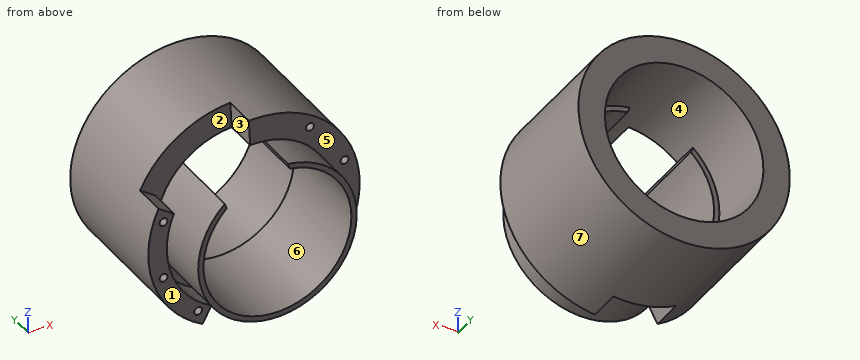
```python
from build123d import *

# Parameters (mm, degrees)
ESBO_O1_R                     = 40
ESBO_O1_R_2                   = 30
RESSALTO_EXTRUS_O1_DEPTH      = 50
ESBO_O2_R                     = 1.5
CORTE_EXTRUS_O1_DEPTH         = 10
CORTE_EXTRUS_O2_DEPTH         = 11.84997677
RESSALTO_EXTRUS_O2_DEPTH      = 26.84997677
RESSALTO_EXTRUS_O2_DEPTH_BACK = 10
ESCALA1_SCALE                 = 0.681818182


with BuildPart() as part:
    # Esboço1 → Ressalto-extrusão1 (new body)
    with BuildSketch(Plane(origin=(0, 0, 0), x_dir=(1, 0, 0), z_dir=(0, 1, 0))):
        with Locations(Location((0, 0, 0), (0, 0, 270))):
            Circle(ESBO_O1_R)
        with Locations(Location((0, 0, 0), (0, 0, 270))):
            Circle(ESBO_O1_R_2, mode=Mode.SUBTRACT)
    extrude(amount=RESSALTO_EXTRUS_O1_DEPTH)

    # Esboço2 → Corte-extrusão1 (cut)
    with BuildSketch(Plane(origin=(0, 0, 0), x_dir=(-1, 0, 0), z_dir=(0, -1, 0))):
        with Locations(Location((-21.160269083, -29.124611797, 0), (0, 0, 90))):
            Circle(ESBO_O2_R)
        with Locations(Location((-34.238034587, -11.124611797, 0), (0, 0, 90))):
            Circle(ESBO_O2_R)
        with Locations(Location((-34.238034587, 11.124611797, 0), (0, 0, 90))):
            Circle(ESBO_O2_R)
        with Locations(Location((21.160269083, 29.124611797, 0), (0, 0, 90))):
            Circle(ESBO_O2_R)
        with Locations(Location((34.238034587, 11.124611797, 0), (0, 0, 90))):
            Circle(ESBO_O2_R)
        with Locations(Location((34.238034587, -11.124611797, 0), (0, 0, 90))):
            Circle(ESBO_O2_R)
    extrude(amount=-CORTE_EXTRUS_O1_DEPTH, mode=Mode.SUBTRACT)

    # Esboço3 → Corte-extrusão2 (cut)
    with BuildSketch(Plane(origin=(0, 0, 0), x_dir=(-1, 0, 0), z_dir=(0, -1, 0))):
        with BuildLine():
            ThreePointArc((30.293924668, -13.087327008), (31.253408489, 10.593604572), (16.092357529, 28.81034587))
            Line((16.092357529, 28.81034587), (19.505887914, 34.921631358))
            ThreePointArc((19.505887914, 34.921631358), (8.030354378, 39.185627576), (-4.197370073, 39.779166463))
            Line((-4.197370073, 39.779166463), (-3.148027555, 29.834374847))
            ThreePointArc((-3.148027555, 29.834374847), (29.911212101, 2.306380417), (1.462902849, -29.964310692))
            Line((1.462902849, -29.964310692), (1.950537132, -39.952414256))
            ThreePointArc((1.950537132, -39.952414256), (22.185986252, -33.283359416), (36.126859334, -17.171197823))
            Line((36.126859334, -17.171197823), (30.293924668, -13.087327008))
        make_face()
    extrude(amount=-CORTE_EXTRUS_O2_DEPTH, mode=Mode.SUBTRACT)

    # Esboço4 → Ressalto-extrusão2 (add, two sides: drawn at the far end of the back side and taken through both)
    with BuildSketch(Plane(origin=(0, 11.84997677, 0), x_dir=(-1, 0, 0), z_dir=(0, -1, 0)).offset(-RESSALTO_EXTRUS_O2_DEPTH_BACK)):
        with BuildLine():
            Line((-4.008838629, -29.730947056), (-4.700362463, -27.602655537))
            ThreePointArc((-4.700362463, -27.602655537), (-8.119302432, 26.79695744), (19.230258499, -20.351834268))
            Line((19.230258499, -20.351834268), (19.909240802, -22.441526924))
            ThreePointArc((19.909240802, -22.441526924), (-8.745833796, 28.696870757), (-4.008838629, -29.730947056))
        make_face()
    extrude(amount=RESSALTO_EXTRUS_O2_DEPTH + RESSALTO_EXTRUS_O2_DEPTH_BACK)


with BuildPart() as part_1:
    # Escala1: scaled about (0, 0, 0)
    add(part.part.scale(ESCALA1_SCALE))


solid = part_1.part
```
Geometry check sheet. Reference: the model listing, model coordinates, mm. Face numbers are marked on the shaded views. A direction names the side the tool comes from. Give positions to 0.01 mm unless a question says otherwise; leave off trailing zeros. Write each loop counter-clockwise with the first axis right and the second up, starting at its lowest first coordinate (ties: lowest second). Pieces come first, ordered by that corner, then holes.
1) Material ranges on L1, parallel to Z at x = -17.5, y = 7; L2, parallel to Z at x = -24, y = 6.5; L3, parallel to Y at x = -23.5, z = -4.5, recorded low to high.
2) Section check B-B, the plane z = 0. Record the boundary of the cut face in (x, y), and give its area (3 significant figures).
3) Release check for a two-part mould opening along Z. For the marked faces 5, 6 and 7 record: pulls with the +Z half, pulls with the -Z half, needs draft (parallel to the pull), parting line crosses it, or undercut.
4) Section check A-A, the plane x = 0. Record the boundary of the cut face in (y, z), and give its area (3 significant figures).
5) Access from +Z, -Z, +X, -X, +Y, -Y to the whole of each face (thin tool, end or side, straight path). Record for the marked faces 1, 2, 3 and 4.
6) Section check D-D, the plane z = -14. Record the boundary of the cut face in (x, y).
7) Section check C-C, the plane y = 4.5. Record the boundary of the cut face in (x, z).
8) Gauge pin test, flat ends, axial feed: pin 1 (1.5 mm diameter, centred on y = 17.5, z = -10.5, fed in from +X); pin 2 (0.6 mm diameter, centred on x = -23, z = 8, fed in from -Y); pin 3 (2 mm diameter, centred on x = 13.5, y = 3, fed in from -Z). Record the tip position at first contact, or that the pin passes through.
Computed:
1. L1: z = -20.92 to -14.14, -10.59 to -7.63, 7.63 to 10.59
1. L2: z = -12.95 to -8.37, -6.8 to 6.8, 8.37 to 11.27
1. L3: y = 0 to 34.09
2. outline: (-27.27, 0) - (-22.5, 0) - (-22.5, 8.08) - (-20.45, 8.08) - (-20.45, -10.23) - (-19.09, -10.23) - (-19.09, 14.9) - (-20.45, 14.9) - (-20.45, 34.09) - (-27.27, 34.09) - close; (19.09, -10.23) - (20.45, -10.23) - (20.45, 0) - (27.27, 0) - (27.27, 34.09) - (20.45, 34.09) - (20.45, 14.9) - (19.09, 14.9) - close
2. area: 517 mm2
3. face 5: needs draft
3. face 6: undercut
3. face 7: parting line crosses it
4. outline: (-10.23, -20.45) - (8.08, -20.45) - (8.08, -27.27) - (34.09, -27.27) - (34.09, -20.45) - (14.9, -20.45) - (14.9, -19.09) - (-10.23, -19.09) - close; (0, 20.45) - (34.09, 20.45) - (34.09, 27.27) - (0, 27.27) - close
4. area: 444 mm2
5. face 1: -Z, -X, -Y
5. face 2: -Y
5. face 3: -X, -Y
5. face 4: +Y
6. outline: (-23.41, 0) - (-17.61, 0) - (-17.61, 8.08) - (-14.91, 8.08) - (-14.91, -10.23) - (-12.98, -10.23) - (-12.98, 14.9) - (-14.91, 14.9) - (-14.91, 34.09) - (-23.41, 34.09) - close; (12.98, -10.23) - (14.91, -10.23) - (14.91, 0) - (23.41, 0) - (23.41, 34.09) - (14.91, 34.09) - (14.91, 14.9) - (12.98, 14.9) - close
7. outline: (-24.63, 11.71) arc R27.27 ccw to (-13.3, -23.81) - (-10.97, -19.64) arc R22.5 cw to (-20.65, 8.92) - close; (-13.57, 15.3) arc R20.45 ccw to (2.15, -20.34) - (2.86, -27.12) arc R27.27 ccw to (-1.33, 27.24) - (-1, 20.43) arc R20.45 cw to (2.73, 20.27) - (3.2, 18.82) arc R19.09 cw (long way) to (-13.11, 13.88) - close; hole circle Ø2.05 at (-23.34, -7.58); hole circle Ø2.05 at (-23.34, 7.58); hole circle Ø2.05 at (-14.43, -19.86); hole circle Ø2.05 at (14.43, 19.86); hole circle Ø2.05 at (23.34, -7.58); hole circle Ø2.05 at (23.34, 7.58)
8. pin 1: stops at x = 25.47
8. pin 2: stops at y = 6.82
8. pin 3: stops at z = -24.24
